Can you work these out from the model? Positions are in its coordinate system, mm. Face numbers are marked on the shaded views. Give positions to 0.01 mm unless a question says otherwise; leave off trailing zeros. Order: outer loops, then holes, each group sorted by start corner. A loop starts at its lowest first (then second) coordinate and runs counter-clockwise, first axis right, second up. Notation, with made-up numbers: M 12,63 L 58,63 A7 cw 58,71 Z; hole C 31.25,54.5 d2. An arc over 180 degrees is marked long. Use a Markdown table: item, result. Add a question column.
from build123d import *

# Parameters (mm, degrees)
SZKIC2_R                    = 7
DODANIE_WYCI_GNI_CIE1_DEPTH = 5
SZKIC5_R                    = 12
DODANIE_WYCI_GNI_CIE3_DEPTH = 15
SZKIC6_R                    = 10
WYTNIJ_WYCI_GNI_CIE1_DEPTH  = 15
SZKIC7_R                    = 3
WYTNIJ_WYCI_GNI_CIE2_DEPTH  = 21.5
SZKIC8_R                    = 3
WYTNIJ_WYCI_GNI_CIE3_DEPTH  = 43


with BuildPart() as part:
    # Szkic2 → Dodanie-wyciągnięcie1 (new body)
    with BuildSketch(Plane.XY):
        with BuildLine():
            Line((130, 7), (1.197449221, 12.944733113))
            ThreePointArc((1.197449221, 12.944733113), (9.606425971, 8.75880015), (13, 0))
            ThreePointArc((13, 0), (9.606425971, -8.75880015), (1.197449221, -12.944733113))
            Line((1.197449221, -12.944733113), (130, -7))
            ThreePointArc((130, -7), (123, 0), (130, 7))
        make_face()
        with Locations((130, 0)):
            Circle(SZKIC2_R)
        with BuildLine():
            Line((1.197449221, 12.944733113), (0, 13))
            ThreePointArc((0, 13), (-13, 0), (0, -13))
            Line((0, -13), (1.197449221, -12.944733113))
            ThreePointArc((1.197449221, -12.944733113), (9.606425971, -8.75880015), (13, 0))
            ThreePointArc((13, 0), (9.606425971, 8.75880015), (1.197449221, 12.944733113))
        make_face()
    extrude(amount=DODANIE_WYCI_GNI_CIE1_DEPTH)

    # Szkic5 → Dodanie-wyciągnięcie3 (add)
    with BuildSketch(Plane.XY.offset(5)):
        Circle(SZKIC5_R)
    extrude(amount=DODANIE_WYCI_GNI_CIE3_DEPTH)

    # Szkic6 → Wytnij-wyciągnięcie1 (cut)
    with BuildSketch(Plane.XY.offset(20)):
        Circle(SZKIC6_R)
    extrude(amount=-WYTNIJ_WYCI_GNI_CIE1_DEPTH, mode=Mode.SUBTRACT)

    # Szkic7 → Wytnij-wyciągnięcie2 (cut, symmetric)
    with BuildSketch(Plane(origin=(0, 0, 0), x_dir=(1, 0, 0), z_dir=(0, 1, 0))):
        with Locations((0, -12.5)):
            Circle(SZKIC7_R)
    extrude(amount=WYTNIJ_WYCI_GNI_CIE2_DEPTH, both=True, mode=Mode.SUBTRACT)

    # Szkic8 → Wytnij-wyciągnięcie3 (cut)
    with BuildSketch(Plane.XY.offset(5)):
        with Locations((130, 0)):
            Circle(SZKIC8_R)
        with Locations((118, 0)):
            Circle(SZKIC8_R)
        with Locations((106, 0)):
            Circle(SZKIC8_R)
        with Locations((94, 0)):
            Circle(SZKIC8_R)
        with Locations((82, 0)):
            Circle(SZKIC8_R)
    extrude(amount=-WYTNIJ_WYCI_GNI_CIE3_DEPTH, mode=Mode.SUBTRACT)


solid = part.part
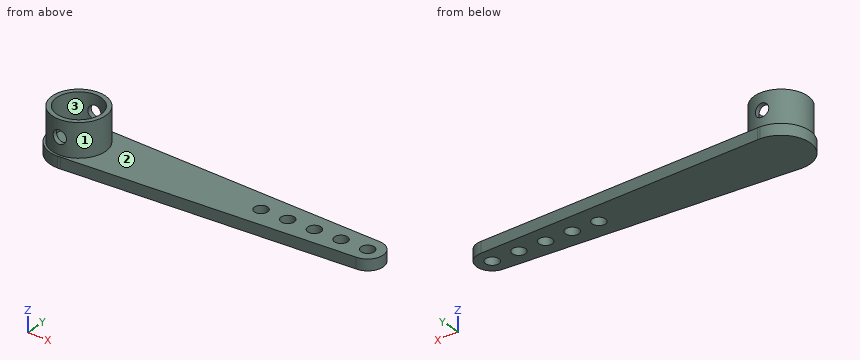
1. If we section it at D-D, the plane x = 39: List the corners of the cut face in (y, z) for me, then the cut area to 3 significant figures.
2. I need wall thicknesses on L1, parallel to X at y = 0.5, z = 15.25; L2, parallel to X at y = 0.25, z = 4.5; L3, parallel to Y at x = 130, z = 2.9. Which ranges of each line are inside material? Lowest first, please. Write a range as [from, to].
3. If we section it at A-A, the plane y = 1.25: State how many separate pieces and enclosed holes the cut face has, then the cut area to 3 significant figures.
4. If we section it at C-C, the plane z = 11: List the corners of the cut face in (x, y) for me, then the cut area to 3 significant figures.
5. If we section it at B-B, the plane x = 82: List the corners of the cut face in (y, z) for me, then the cut area to 3 significant figures.
6. Will these pins go through, and if not, where does the flat tip stop? pin 1 (6 mm diameter, centred on x = 3.5, y = -2, fed in from +Z); pin 2 (9.5 mm diameter, centred on x = 0, z = 12.5, fed in from -Y); pin 3 (1 mm diameter, centred on y = -8, z = 7, fed in from +X); pin 4 (5.5 mm diameter, centred on x = 94, y = 0, fed in from +Z).
7. We'd pull the mould along Y, two halves only. Please class the marked faces 1, 2 and 3: +Y half, -Y half, draft (parallel to the pull), parting line (faces both ways), or undercut.
Geometry results:
| question | item | result |
|---|---|---|
| 1 | outline | M -11.2,0 L 11.2,0 L 11.2,5 L -11.2,5 Z |
| 1 | area | 112 mm^2 |
| 2 | L1 | x = [-11.99, -9.99], [9.99, 11.99] |
| 2 | L2 | x = [-13, 79.01], [84.99, 91.01], [96.99, 103.01], [108.99, 115.01], [120.99, 127.01], [132.99, 137] |
| 2 | L3 | y = [-7, -3], [3, 7] |
| 3 | separate pieces | 6 |
| 3 | enclosed holes | 0 |
| 3 | area | 673 mm^2 |
| 4 | outline | M -2.6,-11.72 L -2.6,-9.66 A10 cw -2.6,9.66 L -2.6,11.72 A12 ccw Z; M 2.6,-11.72 A12 ccw 2.6,11.72 L 2.6,9.66 A10 cw 2.6,-9.66 Z |
| 4 | area | 117 mm^2 |
| 5 | outline | M -9.22,0 L -3,0 L -3,5 L -9.22,5 Z; M 3,0 L 9.22,0 L 9.22,5 L 3,5 Z |
| 5 | area | 62.2 mm^2 |
| 6 | pin 1 | stops at z = 5 |
| 6 | pin 2 | stops at y = -12 |
| 6 | pin 3 | stops at x = 9.37 |
| 6 | pin 4 | passes through |
| 7 | face 1 | parting line |
| 7 | face 2 | draft |
| 7 | face 3 | undercut |
